from build123d import *
from build123d.topology import SkipClean

# Parameters (mm, degrees)
SKETCH_1_R               = 27
EXTRUDE_1_DEPTH          = 10
FILLET_1_R               = 2
SKETCH_2_R               = 15.5
CUT_EXTRUDE_2_DEPTH      = 6
SKETCH_4_R               = 9
EXTRUDE_2_DEPTH          = 5
CUT_EXTRUDE_3_DEPTH      = 10
SKETCH_6_R               = 1.5
CUT_EXTRUDE_4_DEPTH      = 40.736633041
CUT_EXTRUDE_START        = -4
SKETCH_8_R               = 15.5
CUT_EXTRUDE_5_DEPTH      = 4
CUT_EXTRUDE_8_DEPTH      = 41.669398882
SKETCH_10_R              = 1.5
CUT_EXTRUDE_9_DEPTH      = 41.669398882
PATTERN_CIRCULAR_2_COUNT = 6
SKETCH_11_R              = 5
CUT_EXTRUDE_10_DEPTH     = 2
FILLET_2_R               = 1
SKETCH_12_OUTSIDE_W      = 71.788
SKETCH_12_OUTSIDE_H      = 71.788
SKETCH_12_OUTSIDE_R      = 17.5
CUT_EXTRUDE_11_DEPTH     = 20
EXTRUDE_3_DEPTH          = 10
PATTERN_CIRCULAR_3_COUNT = 12
SKETCH_15_R              = 32.027558883
CUT_EXTRUDE_12_DEPTH     = 1
SKETCH_16_R              = 25.808515359
CUT_EXTRUDE_13_DEPTH     = 1


with BuildPart() as part:
    # 草图1 → 凸台-拉伸1 (new, symmetric)
    with BuildSketch(Plane.XY):
        Circle(SKETCH_1_R)
    extrude(amount=EXTRUDE_1_DEPTH, both=True)

    # 圆角1
    fillet_1_edges = [part.edges().sort_by_distance(p)[0] for p in [
        (-27, 0, -10),
        (-27, 0, 10),
    ]]
    fillet(fillet_1_edges, radius=FILLET_1_R)

    # 草图2 → 切除-拉伸2 (cut)
    with BuildSketch(Plane.XY.offset(10)):
        Circle(SKETCH_2_R)
    extrude(amount=-CUT_EXTRUDE_2_DEPTH, mode=Mode.SUBTRACT)

    # 草图4 → 凸台-拉伸2 (add)
    with BuildSketch(Plane.XY.offset(4)):
        Circle(SKETCH_4_R)
    extrude(amount=EXTRUDE_2_DEPTH)

    # 草图5 → 切除-拉伸3 (cut)
    with BuildSketch(Plane.XY.offset(9)):
        Polygon((0, 6.92820323), (-6, 3.464101615), (-6, -3.464101615), (0, -6.92820323), (6, -3.464101615), (6, 3.464101615), align=None)
    extrude(amount=-CUT_EXTRUDE_3_DEPTH, mode=Mode.SUBTRACT)

    # 草图6 → 切除-拉伸4 (cut, through all)
    with BuildSketch(Plane.XY.offset(-1)):
        Circle(SKETCH_6_R)
    extrude(amount=-CUT_EXTRUDE_4_DEPTH, mode=Mode.SUBTRACT)

    # 草图8 → 切除-拉伸5 (cut)
    with BuildSketch(Plane(origin=(0, 0, -10), x_dir=(-1, 0, 0), z_dir=(0, 0, -1)).offset(CUT_EXTRUDE_START)):
        with Locations(Location((0, 0, 0), (0, 0, 180))):
            Circle(SKETCH_8_R)
    extrude(amount=CUT_EXTRUDE_5_DEPTH, mode=Mode.SUBTRACT)

    # 草图9 → 切除-拉伸8 (cut, through all)
    with SkipClean():  # the faces are left unmerged after this step: merging them gives an invalid solid
        with BuildSketch(Plane.XY.offset(4)):
            with BuildLine():
                Line((-8.904732448, 0.5), (-14.57957217, 5.261755918))
                ThreePointArc((-14.57957217, 5.261755918), (-15.5, 0), (-14.57957217, -5.261755918))
                Line((-14.57957217, -5.261755918), (-8.904732448, -0.5))
                ThreePointArc((-8.904732448, -0.5), (-8.91875888, 0), (-8.904732448, 0.5))
            make_face()
        cut_extrude_8 = extrude(amount=-CUT_EXTRUDE_8_DEPTH, mode=Mode.SUBTRACT)
    add(part.part.scale(1), mode=Mode.REPLACE)  # the faces are merged on a copy

    # 草图10 → 切除-拉伸9 (cut, through all)
    with BuildSketch(Plane.XY.offset(4)):
        with Locations((0, 12)):
            Circle(SKETCH_10_R)
    cut_extrude_9 = extrude(amount=-CUT_EXTRUDE_9_DEPTH, mode=Mode.SUBTRACT)

    # 阵列(圆周)2: 切除-拉伸8, 切除-拉伸9 ×6 about axis
    with SkipClean():  # the faces are left unmerged after this step: merging them gives an invalid solid
        pattern_circular_2_axis = Axis((0, 0, 0), (0, 0, 1))
        add([cut_extrude_8.rotate(pattern_circular_2_axis, i * 360 / PATTERN_CIRCULAR_2_COUNT) for i in range(1, PATTERN_CIRCULAR_2_COUNT)], mode=Mode.SUBTRACT)
        add([cut_extrude_9.rotate(pattern_circular_2_axis, i * 360 / PATTERN_CIRCULAR_2_COUNT) for i in range(1, PATTERN_CIRCULAR_2_COUNT)], mode=Mode.SUBTRACT)

    # 草图11 → 切除-拉伸10 (cut)
    with SkipClean():  # the faces are left unmerged after this step: merging them gives an invalid solid
        with BuildSketch(Plane(origin=(0, 0, -6), x_dir=(-1, 0, 0), z_dir=(0, 0, -1))):
            Circle(SKETCH_11_R)
        extrude(amount=-CUT_EXTRUDE_10_DEPTH, mode=Mode.SUBTRACT)

    # 圆角2
    fillet_2_edges = [part.edges().sort_by_distance(p)[0] for p in [
        (5, 0, -6),
    ]]
    fillet(fillet_2_edges, radius=FILLET_2_R)

    # 草图12 outside → 切除-拉伸11 (cut)
    with BuildSketch(Plane.XY.offset(10)):
        Rectangle(SKETCH_12_OUTSIDE_W, SKETCH_12_OUTSIDE_H)
        Circle(SKETCH_12_OUTSIDE_R, mode=Mode.SUBTRACT)
    extrude(amount=-CUT_EXTRUDE_11_DEPTH, mode=Mode.SUBTRACT)

    # 草图13 → 凸台-拉伸3 (add, symmetric)
    with BuildSketch(Plane.XY):
        with BuildLine():
            Line((0.5, 17.492855685), (0.5, 19.5))
            Line((0.5, 19.5), (2, 19.5))
            Line((2, 19.5), (2, 20))
            Line((2, 20), (-2, 20))
            Line((-2, 20), (-2, 19.5))
            Line((-2, 19.5), (-0.5, 19.5))
            Line((-0.5, 19.5), (-0.5, 17.492855685))
            ThreePointArc((-0.5, 17.492855685), (0, 17.5), (0.5, 17.492855685))
        make_face()
    extrude_3 = extrude(amount=EXTRUDE_3_DEPTH, both=True)

    # 阵列(圆周)3: 凸台-拉伸3 ×12 about axis
    with SkipClean():  # the faces are left unmerged after this step: merging them gives an invalid solid
        pattern_circular_3_axis = Axis((0, 0, 0), (0, 0, 1))
        for i in range(1, PATTERN_CIRCULAR_3_COUNT):
            add(extrude_3.rotate(pattern_circular_3_axis, i * 360 / PATTERN_CIRCULAR_3_COUNT))

    # 草图15 → 切除-拉伸12 (cut)
    with SkipClean():  # the faces are left unmerged after this step: merging them gives an invalid solid
        with BuildSketch(Plane(origin=(0, 0, -10), x_dir=(-1, 0, 0), z_dir=(0, 0, -1))):
            Circle(SKETCH_15_R)
        extrude(amount=-CUT_EXTRUDE_12_DEPTH, mode=Mode.SUBTRACT)

    # 草图16 → 切除-拉伸13 (cut)
    with BuildSketch(Plane.XY.offset(10)):
        Circle(SKETCH_16_R)
    extrude(amount=-CUT_EXTRUDE_13_DEPTH, mode=Mode.SUBTRACT)


solid = part.part
The listing builds one solid part. Answer for the finished solid, in the listing's coordinates (mm). A direction names the side the tool comes from. Give positions to 0.01 mm unless a question says otherwise; leave off trailing zeros. Order: outer loops, then holes, each group sorted by start corner. A loop starts at its lowest first (then second) coordinate and runs counter-clockwise, first axis right, second up. Notation, with made-up numbers: (14.25, 23) -> (18.25, 23) arc R18 ccw to (18.25, 42) -> close; hole circle Ø11 at (-36, 45). An arc over 180 degrees is marked (long way). Put each result on its own line as item: value.
Item 1: A cutting plane is placed at A-A on z = 6.25. Count the separate pieces of the cut face and the enclosed holes in it, plus the area to 3 significant figures.
Established:
separate pieces: 2
enclosed holes: 2
area: 385 mm^2
Item 2: Straight lines are drawn through the part: line 1 (Y direction, x = 0, z = -3.3); line 2 (Y direction, x = 0, z = -4.65); line 3 (X direction, y = -15.5, z = 2). For each, find the intervals that lie inside material, in ascending order.
Established:
line 1: y = -20 to -13.5, -10.5 to -1.5, 1.5 to 10.5, 13.5 to 20
line 2: y = -20 to -13.5, -10.5 to -5, 5 to 10.5, 13.5 to 20
line 3: x = -9.53 to -8.37, -8.12 to 8.12, 8.37 to 9.53
Item 3: A cutting plane is placed at B-B on y = -11. Give the vertices of the cut face in (x, z), plus the area to 3 significant figures.
Established:
outline: (-16.74, -9) -> (-16.17, -9) -> (-16.17, 9) -> (-16.74, 9) -> close; (-13.61, -9) -> (-10.92, -9) -> (-10.92, 9) -> (-13.61, 9) -> close; (-3.48, -6) -> (-1.12, -6) -> (-1.12, 4) -> (-3.48, 4) -> close; (1.12, -6) -> (3.48, -6) -> (3.48, 4) -> (1.12, 4) -> close; (10.92, -9) -> (13.61, -9) -> (13.61, 9) -> (10.92, 9) -> close; (16.17, -9) -> (16.74, -9) -> (16.74, 9) -> (16.17, 9) -> close
area: 165 mm^2
Item 4: For faces 4 (the face through (-8.658, -17.518, 0.126)), 5 (the face through (6, 0, 4)), 6 (the face through (-5, 15, 9)), 7 (the face through (8.92, 0.01, -0.93)), determine the directions among +Z, -Z, +X, -X, +Y, -Y from which every point of the face is accessible in a straight line to the end or side of a thin tool.
Established:
face 4: +Z, -Z
face 5: +Z
face 6: +Z, +X, -X, +Y, -Y
face 7: -Z
Item 5: Given P1, Ø5, axis at x = 0, y = -12, coming from the -Z side; P2, Ø10.5, axis at x = 11.5, y = 3.5, coming from the +Z side; P3, Ø4, axis at y = -6.5, z = -1.5, coming from the -X side; P4, Ø6, axis at x = -12, z = 2, coming from the -Y side, each flat-ended and moving along its own axis, determine where each tip first touches the part or whether it passes through.
Established:
P1: stops at z = -6
P2: stops at z = 9
P3: stops at x = -18.32
P4: stops at y = -17.9
Item 6: For a pull along X with two mould halves and no side action, classify faces 1 (the face through (-2, -6, 9)), 2 (the face through (8.677, -17.507, 0.126)), 3 (the face through (-16.28, 8.82, 0.13)) as released by +X, released by -X, zero draft, split by the parting line, or undercut.
Established:
face 1: zero draft
face 2: undercut
face 3: undercut
